Model file for the job. Use its own axes, mm. Round coordinates to 2 decimals unless told otherwise and drop trailing zeros. Order: outer loops, then holes, each group sorted by start corner. A loop starts at its lowest first (then second) coordinate and runs counter-clockwise, first axis right, second up. Notation, with made-up numbers: (33, -19.5) - (61, -19.5) arc R20 ccw to (61, -0.5) - close; hole circle Ø2 at (-4.75, 25.5). An arc over 180 degrees is marked (long way). Write item = value, one per line.
```python
from build123d import *

# Parameters (mm, degrees)
IZIM1_R                          = 0.25
Y_KSEKLIK_EKSTR_ZYON1_DEPTH      = 2.5
IZIM2_R                          = 0.25
Y_KSEKLIK_EKSTR_ZYON2_DEPTH      = 5.5
Y_KSEKLIK_EKSTR_ZYON2_DEPTH_BACK = 5


with BuildPart() as part:
    # Çizim1 → Yükseklik-Ekstrüzyon1 (new body)
    with BuildSketch(Plane(origin=(0, 0, 0), x_dir=(1, 0, 0), z_dir=(0, 1, 0))):
        with BuildLine():
            Line((-2.3, 1.25), (-0.1, 1.25))
            ThreePointArc((-0.1, 1.25), (0, 1.15), (0.1, 1.25))
            Line((0.1, 1.25), (2.3, 1.25))
            ThreePointArc((2.3, 1.25), (2.441421356, 1.191421356), (2.5, 1.05))
            Line((2.5, 1.05), (2.5, -1.05))
            ThreePointArc((2.5, -1.05), (2.441421356, -1.191421356), (2.3, -1.25))
            Line((2.3, -1.25), (0.1, -1.25))
            ThreePointArc((0.1, -1.25), (0, -1.15), (-0.1, -1.25))
            Line((-0.1, -1.25), (-2.3, -1.25))
            ThreePointArc((-2.3, -1.25), (-2.441421356, -1.191421356), (-2.5, -1.05))
            Line((-2.5, -1.05), (-2.5, 1.05))
            ThreePointArc((-2.5, 1.05), (-2.441421356, 1.191421356), (-2.3, 1.25))
        make_face()
        with Locations((-1.25, 0)):
            Circle(IZIM1_R, mode=Mode.SUBTRACT)
        with Locations((1.25, 0)):
            Circle(IZIM1_R, mode=Mode.SUBTRACT)
    extrude(amount=Y_KSEKLIK_EKSTR_ZYON1_DEPTH)

    # Çizim2 → Yükseklik-Ekstrüzyon2 (add, two sides)
    with BuildSketch(Plane(origin=(0, 2.5, 0), x_dir=(1, 0, 0), z_dir=(0, 1, 0))) as y_kseklik_ekstr_zyon2_sk:
        with Locations((-1.25, 0)):
            Circle(IZIM2_R)
        with Locations((1.25, 0)):
            Circle(IZIM2_R)
    extrude(amount=Y_KSEKLIK_EKSTR_ZYON2_DEPTH)
    extrude(y_kseklik_ekstr_zyon2_sk.sketch, amount=-Y_KSEKLIK_EKSTR_ZYON2_DEPTH_BACK)


solid = part.part
```
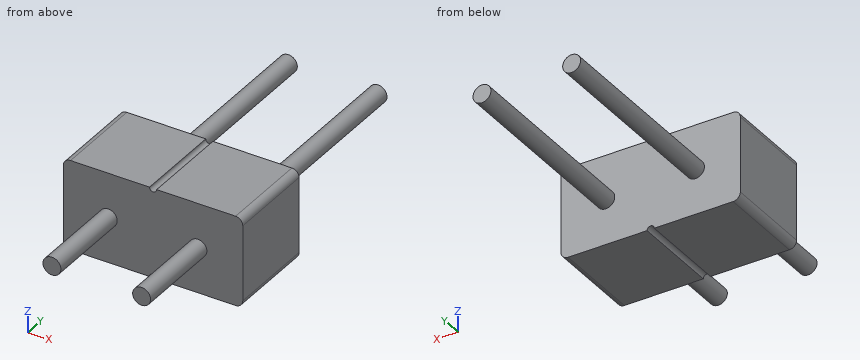
1) Cut at A-A (z = 0). Write the cut outline in (x, y).
Conclusion:
outline = (-2.5, 0) - (-1.5, 0) - (-1.5, -2.5) - (-1, -2.5) - (-1, 0) - (1, 0) - (1, -2.5) - (1.5, -2.5) - (1.5, 0) - (2.5, 0) - (2.5, 2.5) - (1.5, 2.5) - (1.5, 8) - (1, 8) - (1, 2.5) - (-1, 2.5) - (-1, 8) - (-1.5, 8) - (-1.5, 2.5) - (-2.5, 2.5) - close
2) Cut at D-D (x = 0). Write the cut outline in (y, z), and give its area (3 significant figures).
Conclusion:
outline = (0, -1.15) - (2.5, -1.15) - (2.5, 1.15) - (0, 1.15) - close
area = 5.75 mm^2
3) Cut at C-C (x = -1.25). Write the cut outline in (y, z).
Conclusion:
outline = (-2.5, -0.25) - (0, -0.25) - (0, -1.25) - (2.5, -1.25) - (2.5, -0.25) - (8, -0.25) - (8, 0.25) - (2.5, 0.25) - (2.5, 1.25) - (0, 1.25) - (0, 0.25) - (-2.5, 0.25) - close
4) Wall check: line 1 along Y through (x, z) = (-0.5, 1.1); line 2 along X through (y, z) = (-1.5, -0.15); line 3 along Z through (x, y) = (1.3, 3.25). Give the ranges that are in metal, low to high.
Conclusion:
line_1 = 0 to 2.5
line_2 = -1.45 to -1.05, 1.05 to 1.45
line_3 = -0.24 to 0.24
5) Flat gauge pin, fed straight in: pin 1 Ø1.5 at (x, y) = (0, 1) entering from +Z. Where does the tip first touch, or does it go through?
Conclusion:
pin_1 = 1.25
6) Cut at B-B (y = 6.25). Write the cut outline in (x, z).
Conclusion:
outline = circle Ø0.5 at (-1.25, 0); circle Ø0.5 at (1.25, 0)
